Here's the drawing with two shaded views (mm, measured from the low corner). I have some questions. A direction names the side the tool comes from. Give positions to 0.01 mm unless a question says otherwise; leave off trailing zeros. Write each loop counter-clockwise with the first axis right and the second up, starting at its lowest first coordinate (ties: lowest second). Pieces come first, ordered by that corner, then holes.
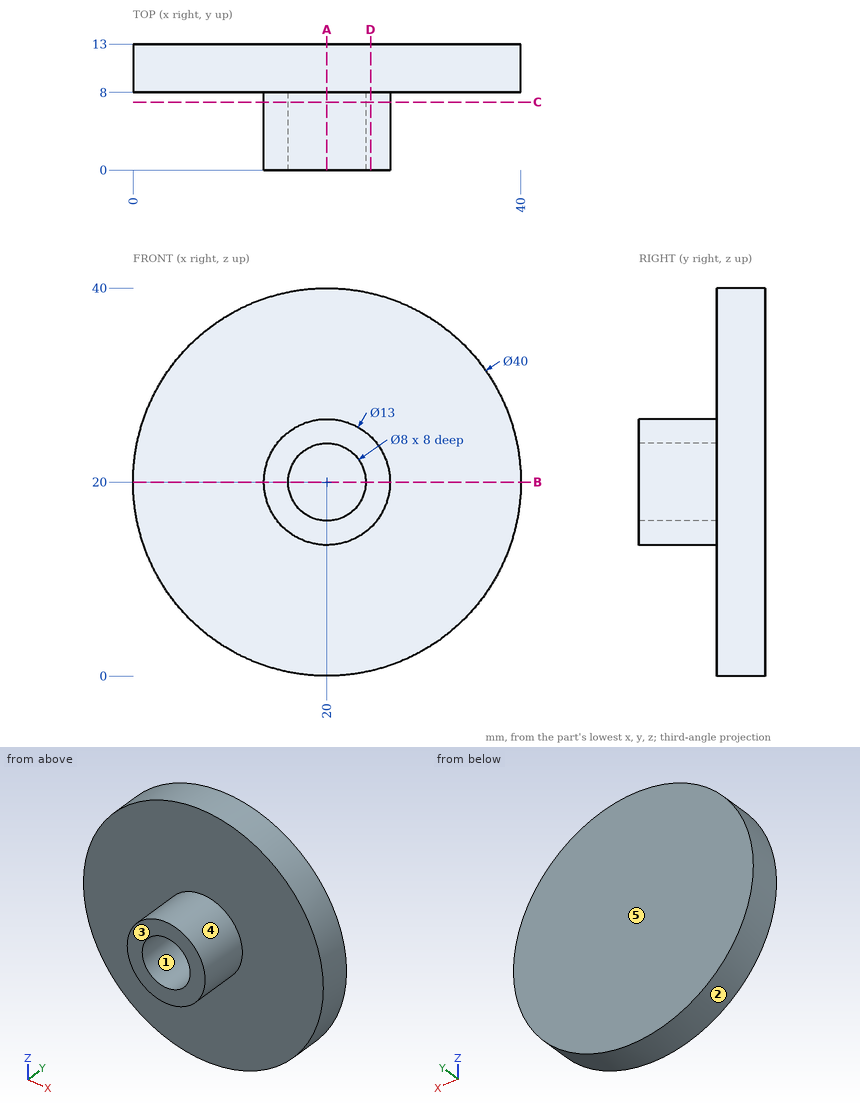
(1) If I drill on L1, parallel to Z at x = 20, y = 5; L2, parallel to Y at x = 28, z = 19; L3, parallel to X at y = 5, z = 23, over which ranges is the centre line in solid material (lowest first)?
Returned:
L1: z = 13.5 to 16, 24 to 26.5
L2: y = 8 to 13
L3: x = 14.23 to 17.35, 22.65 to 25.77
(2) If we mould it in two halves opening along Z, with no side actions, what happens to the marked faces 1, 2 and 3? For each: +Z half, -Z half, draft (parallel to the pull), parting line (faces both ways), or undercut.
Returned:
face 1: undercut
face 2: parting line
face 3: draft
(3) Imagine slicing it at C-C, the plane y = 7. Write out the boundary of the cut face in (x, z).
Returned:
outline: circle Ø13 at (20, 20); hole circle Ø8 at (20, 20)
(4) For the marked faces 4 and 5, which set-ups out of +Z, -Z, +X, -X, +Y, -Y let a thin tool reach every point of the face, with its end or its side?
Returned:
face 4: -Y
face 5: +Z, -Z, +X, -X, +Y
(5) Imagine slicing it at A-A, the plane x = 20. Write out the boundary of the cut face in (y, z).
Returned:
outline: (0, 13.5) - (8, 13.5) - (8, 0) - (13, 0) - (13, 40) - (8, 40) - (8, 26.5) - (0, 26.5) - (0, 24) - (8, 24) - (8, 16) - (0, 16) - close
(6) Will these pins go through, and if not, where does the flat tip stop? P1, Ø6, axis at y = 10, z = 12, coming from the +X side; P2, Ø4, axis at x = 19.5, z = 19, coming from the -Y side; P3, Ø6, axis at x = 15.5, y = 10, coming from the -Z side.
Returned:
P1: stops at x = 39.36
P2: stops at y = 8
P3: stops at z = 0.06
(7) Imagine slicing it at B-B, the plane z = 20. Write out the boundary of the cut face in (x, y), plus the area to 3 significant figures.
Returned:
outline: (0, 8) - (13.5, 8) - (13.5, 0) - (16, 0) - (16, 8) - (24, 8) - (24, 0) - (26.5, 0) - (26.5, 8) - (40, 8) - (40, 13) - (0, 13) - close
area: 240 mm2
(8) Imagine slicing it at D-D, the plane x = 24.5. Write out the boundary of the cut face in (y, z), plus the area to 3 significant figures.
Returned:
outline: (0, 15.31) - (8, 15.31) - (8, 0.51) - (13, 0.51) - (13, 39.49) - (8, 39.49) - (8, 24.69) - (0, 24.69) - close
area: 270 mm2
